Check sheet for the modelled part. Datum: model origin and axes. Units: mm. A direction names the side the tool comes from. Give positions to 0.01 mm unless a question says otherwise; leave off trailing zeros. Loops run counter-clockwise (first coordinate to the right, second up) from the corner with the lowest first, then second, coordinate; pieces in that order, holes last. Notation, with made-up numbers: M -15.75,-7.75 L -11.75,-7.75 A22 cw -11.75,13.25 Z; hole C 24,-22 d7. An arc over 180 degrees is marked long. Use one line per item in the form item = value.
from build123d import *

# Parameters (mm, degrees)
SKETCH2_R           = 7.5
SKETCH2_W           = 9
SKETCH2_H           = 9
BOSS_EXTRUDE1_DEPTH = 10
SKETCH2_4_R         = 5
BOSS_EXTRUDE2_DEPTH = 20
SKETCH3_R           = 2
CUT_EXTRUDE1_DEPTH  = 8.5
SKETCH4_R           = 7.5
BOSS_EXTRUDE3_DEPTH = 1


with BuildPart() as part:
    # Sketch2 → Boss-Extrude1 (new body)
    with BuildSketch(Plane(origin=(0, 0, 0), x_dir=(1, 0, 0), z_dir=(0, 1, 0))):
        Circle(SKETCH2_R)
        Rectangle(SKETCH2_W, SKETCH2_H, mode=Mode.SUBTRACT)
    extrude(amount=BOSS_EXTRUDE1_DEPTH)

    # Sketch2_4 → Boss-Extrude2 (add)
    with BuildSketch(Plane(origin=(0, 0, 0), x_dir=(1, 0, 0), z_dir=(0, 1, 0))):
        Circle(SKETCH2_4_R)
    extrude(amount=-BOSS_EXTRUDE2_DEPTH)

    # Sketch3 → Cut-Extrude1 (cut)
    with BuildSketch(Plane.XZ.offset(20)):
        Circle(SKETCH3_R)
    extrude(amount=-CUT_EXTRUDE1_DEPTH, mode=Mode.SUBTRACT)

    # Sketch4 → Boss-Extrude3 (add)
    with BuildSketch(Plane.XZ):
        Circle(SKETCH4_R)
    extrude(amount=BOSS_EXTRUDE3_DEPTH)


solid = part.part
1) Section check D-D (y = -3.5). Record the cut outline in (x, z), then the cut area to 3 significant figures.
Evaluation:
outline = C 0,0 d10
area = 78.5 mm^2
2) Section check A-A (y = 7.5). Record the cut outline in (x, z).
Evaluation:
outline = C 0,0 d15; hole M -4.5,-4.5 L 4.5,-4.5 L 4.5,4.5 L -4.5,4.5 Z
3) Release check for a two-part mould opening along X. For faces 1 (the face through (-4.5, 5, 0)), 2 (the face through (-7.493, 4.577, 0.33)), 3 (the face through (0, 10, 5)) record: pulls with the +X half, pulls with the -X half, needs draft (parallel to the pull), parting line crosses it, or undercut.
Evaluation:
face_1 = undercut
face_2 = parting line crosses it
face_3 = needs draft
4) Section check B-B (x = 0). Record the cut outline in (y, z).
Evaluation:
outline = M -20,-5 L -1,-5 L -1,-7.5 L 10,-7.5 L 10,-4.5 L 0,-4.5 L 0,4.5 L 10,4.5 L 10,7.5 L -1,7.5 L -1,5 L -20,5 L -20,2 L -11.5,2 L -11.5,-2 L -20,-2 Z
5) Set-up check for faces 4 (the face through (4.5, 5, 0)), 5 (the face through (-1.08, -10.37, 4.88)), 6 (the face through (-0.1, -20, 2.2)): record each of +Z, -Z, +X, -X, +Y, -Y from which the full face is reachable in a straight line by a thin tool's end or side.
Evaluation:
face_4 = +Y
face_5 = -Y
face_6 = +Z, -Z, +X, -X, -Y
6) Section check C-C (z = 0). Record the cut outline in (x, y).
Evaluation:
outline = M -7.5,-1 L -5,-1 L -5,-20 L -2,-20 L -2,-11.5 L 2,-11.5 L 2,-20 L 5,-20 L 5,-1 L 7.5,-1 L 7.5,10 L 4.5,10 L 4.5,0 L -4.5,0 L -4.5,10 L -7.5,10 Z
7) Scan lines: line 1 (Z direction, x = 0, y = -16); line 2 (X direction, y = 0.5, z = -6); line 3 (Y direction, x = 0, z = -1.5). Record each from-to range of solid material in increasing order.
Evaluation:
line_1 = -5 to -2, 2 to 5
line_2 = -4.5 to 4.5
line_3 = -11.5 to 0
8) Depth check by flat-ended pin: pin 1 Ø5 at (y, z) = (-7, 5.5) entering from +X; pin 2 Ø2 at (y, z) = (-7, 4.5) entering from +X; pin 3 Ø1.5 at (x, y) = (5, 0.5) entering from -Z. Enter the tip coordinate at first touch or a pass-through.
Evaluation:
pin_1 = 4
pin_2 = 3.57
pin_3 = -6.18
